Geometry: final body of the model. Coordinates: model frame, mm. A direction names the side the tool comes from. Give positions to 0.01 mm unless a question says otherwise; leave off trailing zeros. Order: outer loops, then holes, each group sorted by start corner. A loop starts at its lowest first (then second) coordinate and runs counter-clockwise, first axis right, second up. Notation, with made-up numbers: M 80,-19.75 L 105,-19.75 A21 ccw 105,10.25 Z; hole C -30,65.5 d6. An arc over 180 degrees is marked long. One line per item, written item: value. Start each with the question number.
```python
from build123d import *

# Parameters (mm, degrees)
SKETCH1_R           = 1.905
SKETCH1_R_2         = 3.175
BOSS_EXTRUDE1_DEPTH = 4.318


with BuildPart() as part:
    # Sketch1 → Boss-Extrude1 (new body)
    with BuildSketch(Plane.XY):
        with BuildLine():
            ThreePointArc((-6.74251391, 12.955482668), (-4.633472823, 17.399161687), (0, 19.05))
            ThreePointArc((0, 19.05), (4.633472823, 17.399161687), (6.74251391, 12.955482668))
            ThreePointArc((6.74251391, 12.955482668), (5.682842224, 10.643577378), (4.397291681, 8.449227827))
            ThreePointArc((4.397291681, 8.449227827), (4.490128061, 4.490128061), (8.449227827, 4.397291681))
            ThreePointArc((8.449227827, 4.397291681), (10.643577378, 5.682842224), (12.955482668, 6.74251391))
            ThreePointArc((12.955482668, 6.74251391), (17.399161687, 4.633472823), (19.05, 0))
            ThreePointArc((19.05, 0), (17.399161687, -4.633472823), (12.955482668, -6.74251391))
            ThreePointArc((12.955482668, -6.74251391), (10.643577378, -5.682842224), (8.449227827, -4.397291681))
            ThreePointArc((8.449227827, -4.397291681), (4.490128061, -4.490128061), (4.397291681, -8.449227827))
            ThreePointArc((4.397291681, -8.449227827), (5.682842224, -10.643577378), (6.74251391, -12.955482668))
            ThreePointArc((6.74251391, -12.955482668), (4.633472823, -17.399161687), (0, -19.05))
            ThreePointArc((0, -19.05), (-4.633472823, -17.399161687), (-6.74251391, -12.955482668))
            ThreePointArc((-6.74251391, -12.955482668), (-5.682842224, -10.643577378), (-4.397291681, -8.449227827))
            ThreePointArc((-4.397291681, -8.449227827), (-4.490128061, -4.490128061), (-8.449227827, -4.397291681))
            ThreePointArc((-8.449227827, -4.397291681), (-10.643577378, -5.682842224), (-12.955482668, -6.74251391))
            ThreePointArc((-12.955482668, -6.74251391), (-17.399161687, -4.633472823), (-19.05, 0))
            ThreePointArc((-19.05, 0), (-17.399161687, 4.633472823), (-12.955482668, 6.74251391))
            ThreePointArc((-12.955482668, 6.74251391), (-10.643577378, 5.682842224), (-8.449227827, 4.397291681))
            ThreePointArc((-8.449227827, 4.397291681), (-4.490128061, 4.490128061), (-4.397291681, 8.449227827))
            ThreePointArc((-4.397291681, 8.449227827), (-5.682842224, 10.643577378), (-6.74251391, 12.955482668))
        make_face()
        with Locations((0, 14.605)):
            Circle(SKETCH1_R, mode=Mode.SUBTRACT)
        with Locations((14.605, 0)):
            Circle(SKETCH1_R, mode=Mode.SUBTRACT)
        with Locations((0, -14.605)):
            Circle(SKETCH1_R, mode=Mode.SUBTRACT)
        with Locations((-14.605, 0)):
            Circle(SKETCH1_R, mode=Mode.SUBTRACT)
        Circle(SKETCH1_R_2, mode=Mode.SUBTRACT)
    extrude(amount=BOSS_EXTRUDE1_DEPTH)


solid = part.part
```
Q1. Set-up query: faces 4 (the face through (5.666, -10.612, 2.129)), 5 (the face through (10.68, -5.7, 2.13)), 6 (the face through (-5.666, 10.612, 2.129)). Return all of +Z, -Z, +X, -X, +Y, -Y with unobstructed straight access to the full face (end or side cutting, diameter ignored); none if empty.
Q2. Section query D-D on y = 10. Return loops of the section in (x, z).
Q3. Section query B-B on z = 0.5. Return loops of the section in (x, y) (3 decimals), and give its area (3 significant figures).
Q4. Mould query, pull axis X, two halves, no side actions, for faces 1 (the face through (-4, 0, 4.318)), 2 (the face through (17.446, -4.581, 2.129)), 3 (the face through (4.53, -4.45, 2.13)). Classes: +X half, -X half, draft (parallel to the pull), parting line (faces both ways), or undercut.
Q5. Ray query, line 1 along Y through (x, z) = (-6, 0.75); line 2 along X through (y, z) = (4.5, 1.85); line 3 along X through (y, z) = (-5, 4.1). Return the intervals inside material, ascending. Write a range as [from, to].
Q6. Section query A-A on x = 5.5. Return loops of the section in (y, z).
Q7. Contact query for flat-ended pins moving along their axis: pin 1 (2 mm diameter, centred on x = 8, z = 3, fed in from -Y); pin 2 (3.5 mm diameter, centred on x = 0, y = -14.605, fed in from +Z); pin 3 (2 mm diameter, centred on x = 11, z = 0.5, fed in from +Y). Output: stop coordinate, or through.
Q8. Section query C-C on x = 13.5. Return loops of the section in (y, z), and give its area (3 significant figures).
Results below:
1. face 4: +Z, -Z, +X
1. face 5: +Z, -Z, -Y
1. face 6: +Z, -Z, -X
2. outline: M -5.34,0 L 5.34,0 L 5.34,4.32 L -5.34,4.32 Z
3. outline: M -19.05,0 A6.427 ccw -12.955,-6.743 A25.4 ccw -8.449,-4.397 A2.868 cw -4.397,-8.449 A25.4 ccw -6.743,-12.955 A6.427 ccw 0,-19.05 A6.427 ccw 6.743,-12.955 A25.4 ccw 4.397,-8.449 A2.868 cw 8.449,-4.397 A25.4 ccw 12.955,-6.743 A6.427 ccw 19.05,0 A6.427 ccw 12.955,6.743 A25.4 ccw 8.449,4.397 A2.868 cw 4.397,8.449 A25.4 ccw 6.743,12.955 A6.427 ccw 0,19.05 A6.427 ccw -6.743,12.955 A25.4 ccw -4.397,8.449 A2.868 cw -8.449,4.397 A25.4 ccw -12.955,6.743 A6.427 ccw Z; hole C -14.605,0 d3.81; hole C 0,0 d6.35; hole C 0,-14.605 d3.81; hole C 0,14.605 d3.81; hole C 14.605,0 d3.81
3. area: 590 mm2
4. face 1: draft
4. face 2: +X half
4. face 3: undercut
5. line 1: [-15.65, -11.27], [-3.7, 3.7], [11.27, 15.65]
5. line 2: [-17.52, -8.61], [-4.48, 4.48], [8.61, 17.52]
5. line 3: [-17.04, -9.42], [-4.08, 4.08], [9.42, 17.04]
6. outline: M -16.44,0 L -10.3,0 L -10.3,4.32 L -16.44,4.32 Z; M -3.84,0 L 3.84,0 L 3.84,4.32 L -3.84,4.32 Z; M 10.3,0 L 16.44,0 L 16.44,4.32 L 10.3,4.32 Z
7. pin 1: y = -4.75
7. pin 2: through
7. pin 3: y = 6.34
8. outline: M -6.69,0 L -1.55,0 L -1.55,4.32 L -6.69,4.32 Z; M 1.55,0 L 6.69,0 L 6.69,4.32 L 1.55,4.32 Z
8. area: 44.4 mm2
